Geometry check sheet. Reference: drawing and pictorial views, mm from the part's lowest x, y, z. A direction names the side the tool comes from. Coordinates: 2 decimals unless noted, no trailing zeros. Write each loop counter-clockwise with the first axis right and the second up, starting at its lowest first coordinate (ties: lowest second). Pieces come first, ordered by that corner, then holes. Notation, with made-up numbers: (81, 56.5) -> (104, 56.5) arc R26 ccw to (104, 72.5) -> close; hole circle Ø6 at (47, 41). An arc over 180 degrees is marked (long way). Answer in a Markdown table with one row per item.
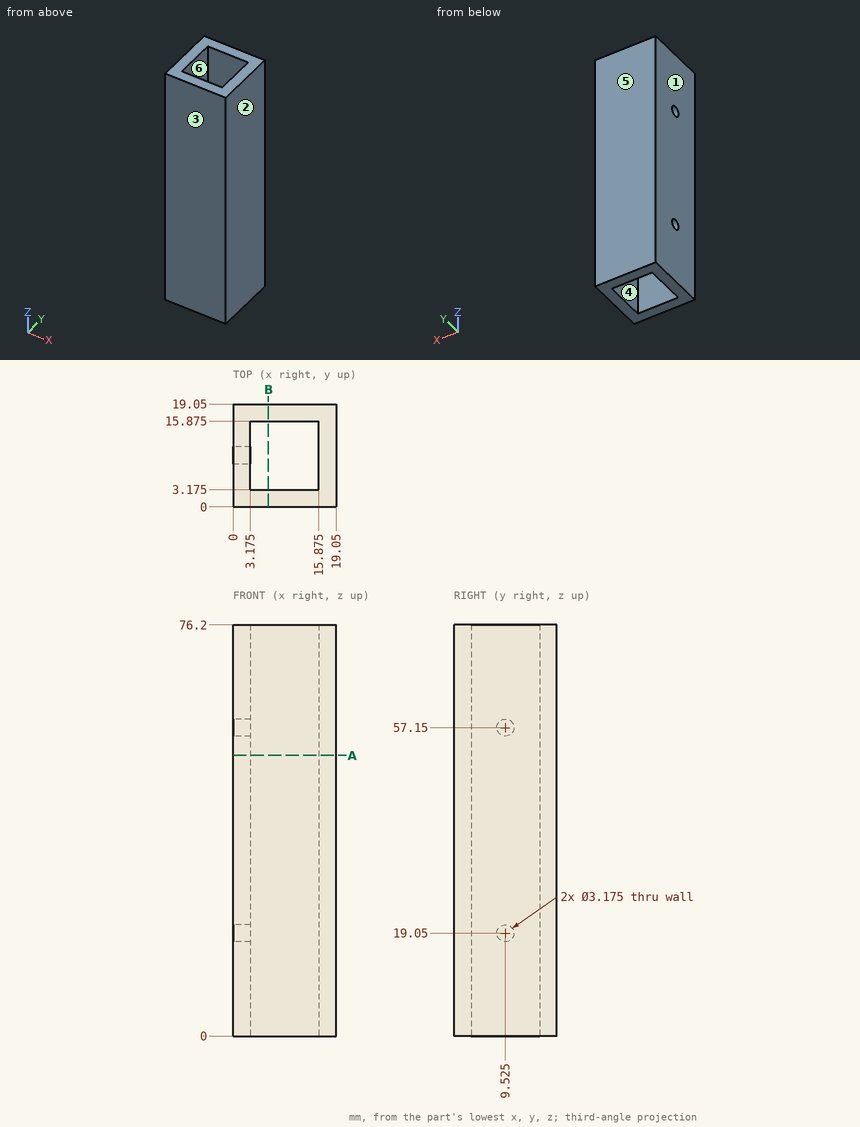
1. Section check B-B, the plane x = 6.5. Record the boundary of the cut face in (y, z) (3 decimals).
Geometry says:
| item | result |
|---|---|
| outline | (0, 0) -> (3.175, 0) -> (3.175, 76.2) -> (0, 76.2) -> close; (15.875, 0) -> (19.05, 0) -> (19.05, 76.2) -> (15.875, 76.2) -> close |
2. Tool access check on the marked faces 5 and 6. Record the directions out of +Z, -Z, +X, -X, +Y, -Y that give a thin tool (end or side, any length) a straight path to the whole face; none if there is none.
Geometry says:
| item | result |
|---|---|
| face 5 | +Z, -Z, +X, -X, +Y |
| face 6 | +Z, -Z |
3. Section check A-A, the plane z = 52. Record the boundary of the cut face in (x, y) (3 decimals).
Geometry says:
| item | result |
|---|---|
| outline | (0, 0) -> (19.05, 0) -> (19.05, 19.05) -> (0, 19.05) -> close; hole (3.175, 3.175) -> (15.875, 3.175) -> (15.875, 15.875) -> (3.175, 15.875) -> close |
4. Thickness scan on line 1 (X direction, y = 9, z = 35) (3 decimals). Record the ranges inside material, lowest first. Write a range as from..to.
Geometry says:
| item | result |
|---|---|
| line 1 | 0..3.175, 15.875..19.05 |
5. Mould release check, pull along X, two halves, no side actions. Record for the marked faces 1, 2, 3 and 4: released by +X, released by -X, zero draft, split by the parting line, or undercut.
Geometry says:
| item | result |
|---|---|
| face 1 | released by -X |
| face 2 | released by +X |
| face 3 | zero draft |
| face 4 | undercut |
6. Depth check by flat-ended pin: P1, Ø1, axis at x = 13, y = 5, coming from the +Z side. Enter the tip coordinate at first touch or a pass-through.
Geometry says:
| item | result |
|---|---|
| P1 | through |
